CAD build for the part. Positions are in the model's coordinates, mm. A direction names the side the tool comes from. Coordinates: 2 decimals unless noted, no trailing zeros. Order: outer loops, then holes, each group sorted by start corner. A loop starts at its lowest first (then second) coordinate and runs counter-clockwise, first axis right, second up. Notation, with made-up numbers: M 3,85.5 L 22,85.5 A25 ccw 22,115.5 Z; hole C -24,-37 d5. An arc over 180 degrees is marked long. One line per item, written item: value.
from build123d import *

# Parameters (mm, degrees)
F0_W     = 111
F0_H     = 65
F1_DEPTH = 5
F2_W     = 103
F2_H     = 57
F3_DEPTH = 50
F4_R     = 2


with BuildPart() as f1:
    # F0 (on Top) → F1 (new body)
    with BuildSketch(Plane.XY):
        Rectangle(F0_W, F0_H)
    extrude(amount=F1_DEPTH)

    # F2 (on Top) → F3 (join)
    with BuildSketch(Plane.XY):
        Rectangle(F2_W, F2_H)
    extrude(amount=-F3_DEPTH)

    # F4
    f4_edges = [f1.edges().sort_by_distance(p)[0] for p in [
        (0, -32.5, 5),
        (55.5, 0, 5),
        (0, 32.5, 5),
        (-55.5, 0, 5),
        (-55.5, 32.5, 2.5),
        (55.5, 32.5, 2.5),
        (55.5, -32.5, 2.5),
        (-55.5, -32.5, 2.5),
    ]]
    fillet(f4_edges, radius=F4_R)


solid = f1.part
Q1. Slice it at A-A (y = -13). List the corners of the cut face in (x, z).
Recorded:
outline: M -55.5,0 L -51.5,0 L -51.5,-50 L 51.5,-50 L 51.5,0 L 55.5,0 L 55.5,3 A2 ccw 53.5,5 L -53.5,5 A2 ccw -55.5,3 Z
Q2. Pin check, flat tips, straight feed: pin 1 Ø5 at (x, z) = (-37.5, -39.5) entering from -Y; pin 2 Ø25 at (y, z) = (-12.5, -21.5) entering from +X; pin 3 Ø2 at (x, z) = (15.5, -34.5) entering from +Y. Stop position of each tip, or through.
Recorded:
pin 1: stops at y = -28.5
pin 2: stops at x = 51.5
pin 3: stops at y = 28.5
Q3. Which spindle directions (+Z, -Z, +X, -X, +Y, -Y) get a long thin tool onto all of the face, cutting with end or side? Do faces 1 (the face through (-1, 28.5, -25)), 2 (the face through (-1, 32.5, 1)), 3 (the face through (-1, -28.5, -25)), 4 (the face through (-51.5, 0, -25)), 5 (the face through (51.5, 0, -25)). Say none if no direction does.
Recorded:
face 1: -Z, +X, -X, +Y
face 2: +Z, -Z, +X, -X, +Y
face 3: -Z, +X, -X, -Y
face 4: -Z, -X, +Y, -Y
face 5: -Z, +X, +Y, -Y
Q4. Slice it at B-B (x = 43). List the corners of the cut face in (y, z).
Recorded:
outline: M -32.5,0 L -28.5,0 L -28.5,-50 L 28.5,-50 L 28.5,0 L 32.5,0 L 32.5,3 A2 ccw 30.5,5 L -30.5,5 A2 ccw -32.5,3 Z
Q5. Drill centre lines: line 1 along Y through (x, z) = (-5, -11); line 2 along X through (y, z) = (13.5, -12.5); line 3 along Z through (x, y) = (24, 29). Where is each one in solid material? Low to high.
Recorded:
line 1: y = -28.5 to 28.5
line 2: x = -51.5 to 51.5
line 3: z = 0 to 5
Q6. Slice it at C-C (z = -2). List the corners of the cut face in (x, y).
Recorded:
outline: M -51.5,-28.5 L 51.5,-28.5 L 51.5,28.5 L -51.5,28.5 Z
